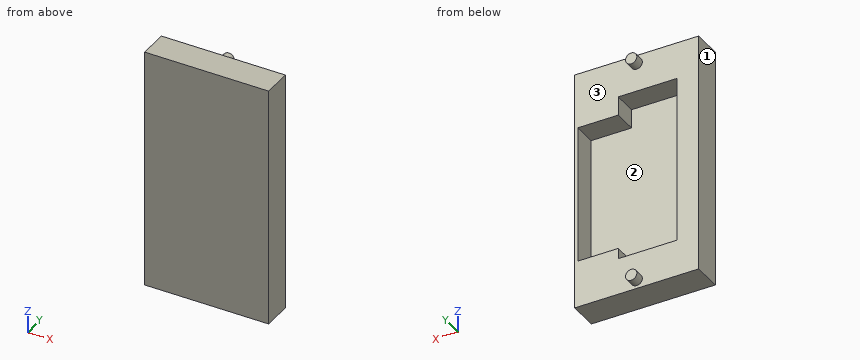
```python
from build123d import *

# Parameters (mm, degrees)
CROQUIS1_W              = 45
CROQUIS1_H              = 75
SALIENTE_EXTRUIR1_DEPTH = 9
CROQUIS2_W              = 18.1
CROQUIS2_H              = 52.1
CROQUIS2_W_2            = 12.5
CROQUIS2_H_2            = 42.938951505
CORTAR_EXTRUIR9_DEPTH   = 7.2
CROQUIS3_W              = 6.70437092
CROQUIS3_H              = 75
CORTAR_EXTRUIR10_DEPTH  = 9
CROQUIS4_R              = 1.745
CROQUIS4_R_2            = 1.75
SALIENTE_EXTRUIR2_DEPTH = 3


with BuildPart() as part:
    # Croquis1 → Saliente-Extruir1 (new body)
    with BuildSketch(Plane(origin=(0, 0, 0), x_dir=(1, 0, 0), z_dir=(0, 1, 0))):
        Rectangle(CROQUIS1_W, CROQUIS1_H)
    extrude(amount=SALIENTE_EXTRUIR1_DEPTH)

    # Croquis2 → Cortar-Extruir9 (cut)
    with BuildSketch(Plane(origin=(0, 9, 0), x_dir=(1, 0, 0), z_dir=(0, 1, 0))):
        Rectangle(CROQUIS2_W, CROQUIS2_H)
        with Locations((15.3, 1.284934341)):
            Rectangle(CROQUIS2_W_2, CROQUIS2_H_2)
    extrude(amount=-CORTAR_EXTRUIR9_DEPTH, mode=Mode.SUBTRACT)

    # Croquis3 → Cortar-Extruir10 (cut)
    with BuildSketch(Plane(origin=(0, 9, 0), x_dir=(1, 0, 0), z_dir=(0, 1, 0))):
        with Locations((-19.14781454, 0)):
            Rectangle(CROQUIS3_W, CROQUIS3_H)
    extrude(amount=-CORTAR_EXTRUIR10_DEPTH, mode=Mode.SUBTRACT)

    # Croquis4 → Saliente-Extruir2 (add)
    with BuildSketch(Plane(origin=(0, 9, 0), x_dir=(1, 0, 0), z_dir=(0, 1, 0))):
        with Locations((3.35218546, -34.85)):
            Circle(CROQUIS4_R)
        with Locations((3.35218546, 34.85)):
            Circle(CROQUIS4_R_2)
    extrude(amount=SALIENTE_EXTRUIR2_DEPTH)


solid = part.part
```
Input: part model. Units: mm. Frame: model coordinates. Face numbers are marked on the shaded views. Coordinates: 2 decimals unless noted, no trailing zeros. Loops run counter-clockwise (first coordinate to the right, second up) from the corner with the lowest first, then second, coordinate; pieces in that order, holes last. Notation, with made-up numbers: M 72.25,51.25 L 124.25,51.25 A17 ccw 124.25,55.25 Z; hole C -12.5,22.5 d10. An arc over 180 degrees is marked long. Answer in a Markdown table with one row per item.
1. Section C-C, the plane z = 34.85. Output: boundary loops of the cut face in (x, y).
Response:
| item | result |
|---|---|
| outline | M -15.8,0 L 22.5,0 L 22.5,9 L 5.1,9 L 5.1,12 L 1.61,12 L 1.61,9 L -15.8,9 Z |
2. Section A-A, the plane y = 8. Output: boundary loops of the cut face in (x, z).
Response:
| item | result |
|---|---|
| outline | M -15.8,-37.5 L 22.5,-37.5 L 22.5,37.5 L -15.8,37.5 Z; hole M -9.05,-26.05 L 9.05,-26.05 L 9.05,-22.75 L 21.55,-22.75 L 21.55,20.18 L 9.05,20.18 L 9.05,26.05 L -9.05,26.05 Z |
3. Section B-B, the plane x = 16. Output: boundary loops of the cut face in (y, z), then the cut area to 3 significant figures.
Response:
| item | result |
|---|---|
| outline | M 0,-37.5 L 9,-37.5 L 9,-22.75 L 1.8,-22.75 L 1.8,20.18 L 9,20.18 L 9,37.5 L 0,37.5 Z |
| area | 366 mm2 |
4. Draft query along X for the marked faces 1, 2 and 3. Return one class per face: pulls with the +X half, pulls with the -X half, needs draft (parallel to the pull), parting line crosses it, or undercut.
Response:
| item | result |
|---|---|
| face 1 | pulls with the -X half |
| face 2 | undercut |
| face 3 | needs draft |
5. First-contact query: pin 1 (12 mm diameter, centred on x = -1, z = 15.5, fed in from +Y); pin 2 (3 mm diameter, centred on x = -10, z = 9, fed in from +Y). Flat tips, straight axial feed; report the tip coordinate or a pass-through.
Response:
| item | result |
|---|---|
| pin 1 | stops at y = 1.8 |
| pin 2 | stops at y = 9 |
6. Section D-D, the plane x = 3. Output: boundary loops of the cut face in (y, z), then the cut area to 3 significant figures.
Response:
| item | result |
|---|---|
| outline | M 0,-37.5 L 9,-37.5 L 9,-36.56 L 12,-36.56 L 12,-33.14 L 9,-33.14 L 9,-26.05 L 1.8,-26.05 L 1.8,26.05 L 9,26.05 L 9,33.14 L 12,33.14 L 12,36.56 L 9,36.56 L 9,37.5 L 0,37.5 Z |
| area | 320 mm2 |
7. Material intervals for line 1 (X direction, y = 3.25, z = -7); line 2 (Z direction, x = 1, y = 2.5); line 3 (Y direction, x = 5.5, z = -11), sorted ascending.
Response:
| item | result |
|---|---|
| line 1 | x = -15.8 to -9.05, 21.55 to 22.5 |
| line 2 | z = -37.5 to -26.05, 26.05 to 37.5 |
| line 3 | y = 0 to 1.8 |
